Model file for the job. Use its own axes, mm. Face numbers are marked on the shaded views. A direction names the side the tool comes from. Coordinates: 2 decimals unless noted, no trailing zeros. Write each loop counter-clockwise with the first axis right and the second up, starting at its lowest first coordinate (ties: lowest second). Pieces come first, ordered by that corner, then holes.
Q1. Band-saw the part on D-D, the plane x = -7.55. Write the cut outline in (y, z) (3 decimals), plus the area to 3 significant figures.
Q2. Drill centre lines: probe 1 along Z at (x, y) = (-7.55, 17.25) (3 decimals); probe 2 along Z at (x, y) = (6.45, 26); probe 3 along X at (y, z) = (41.5, 45.6) (3 decimals). Where is each one in solid material? Low to high.
Q3. Which spindle directions (+Z, -Z, +X, -X, +Y, -Y) get a long thin tool onto all of the face, cutting with end or side? Do the marked faces 1, 2, 3 and 4. Say none if no direction does.
Q4. Pin check, flat tips, straight feed: P1, Ø16.5, axis at y = 27, z = 12, coming from the -X side; P2, Ø1.9, axis at y = 6, z = 31, coming from the -X side; P3, Ø4, axis at x = -7.55, z = 7, coming from the +Y side. Stop position of each tip, or through.
Q5. Band-saw the part on A-A, the plane x = 23. Write the cut outline in (y, z), plus the area to 3 significant figures.
Q6. Band-saw the part on B-B, the plane y = 26. Write the cut outline in (x, z) (3 decimals), plus the area to 3 significant figures.
Q7. Pull direction Z, two halves, no side cores. Call the marked faces 5, 6 and 7: released by +Z, released by -Z, zero draft, split by the parting line, or undercut.
from build123d import *

# Parameters (mm, degrees)
F0_W      = 10
F0_H      = 52
F1_DEPTH  = 44
F2_W      = 54
F2_H      = 52
F3_DEPTH  = 4
F5_DEPTH  = 4
F7_DEPTH  = 4
F8_R      = 15
F8_R_2    = 1.725
F9_DEPTH  = 4
F10_R     = 1.725
F11_DEPTH = 10
F10_R_2   = 3.5
F12_DEPTH = 6
F14_W     = 15.1
F14_H     = 4
F15_DEPTH = 48
F16_R     = 1.725
F17_DEPTH = 4
F18_R     = 1.725
F19_DEPTH = 4
F20_R     = 4
F21_R     = 1.99999


# Not quite as in the source:
# - a fillet or chamfer is up to 0.001 mm smaller than in the source, because OpenCascade refuses the exact size
# - a feature of the source that left no trace in its solid (it failed there, or was rolled back) is left out
# - a feature names something its author has since deleted; it is built from what else it names


with BuildPart() as f1:
    # F0 (on Top) → F1 (new body)
    with BuildSketch(Plane.XY):
        with Locations((5, 26)):
            Rectangle(F0_W, F0_H)
    extrude(amount=F1_DEPTH)

    # F2 (on face) → F3 (join)
    with BuildSketch(Plane.XY.offset(44)):
        with Locations((27, 26)):
            Rectangle(F2_W, F2_H)
    extrude(amount=F3_DEPTH)

    # F4 (on face) → F5 (join)
    with BuildSketch(Plane.XZ):
        Polygon((10, 0), (54, 44), (10, 44), align=None)
    extrude(amount=-F5_DEPTH)

    # F6 (on face) → F7 (join)
    with BuildSketch(Plane(origin=(0, 52, 0), x_dir=(-1, 0, 0), z_dir=(0, 1, 0))):
        Polygon((-10, 44), (-54, 44), (-10, 0), align=None)
    extrude(amount=-F7_DEPTH)

    # F8 (on face) → F9 (cut, through all)
    with BuildSketch(Plane(origin=(0, 0, 44), x_dir=(1, 0, 0), z_dir=(0, 0, -1))):
        with Locations((32, -26)):
            Circle(F8_R)
        with Locations((16.5, -10.5)):
            Circle(F8_R_2)
        with Locations((47.5, -10.5)):
            Circle(F8_R_2)
        with Locations((47.5, -41.5)):
            Circle(F8_R_2)
        with Locations((16.5, -41.5)):
            Circle(F8_R_2)
    extrude(amount=-F9_DEPTH, mode=Mode.SUBTRACT)

    # F10 (on face) → F11 (cut)
    with BuildSketch(Plane.YZ.offset(10)):
        with Locations((26, 37)):
            Circle(F10_R)
        with Locations((26, 7)):
            Circle(F10_R)
    extrude(amount=-F11_DEPTH, mode=Mode.SUBTRACT)

    # F10 (on face) → F12 (cut)
    with BuildSketch(Plane.YZ.offset(10)):
        with Locations((26, 37)):
            Circle(F10_R_2)
        with Locations((26, 37)):
            Circle(F10_R, mode=Mode.SUBTRACT)
        with Locations((26, 7)):
            Circle(F10_R_2)
        with Locations((26, 7)):
            Circle(F10_R, mode=Mode.SUBTRACT)
    extrude(amount=-F12_DEPTH, mode=Mode.SUBTRACT)

    # F14 (on face) → F15 (join)
    with BuildSketch(Plane.XY.offset(48)):
        with Locations((-7.55, 35.55)):
            Rectangle(F14_W, F14_H)
        with Locations((-7.55, 16.45)):
            Rectangle(F14_W, F14_H)
    extrude(amount=-F15_DEPTH)

    # F16 (on face) → F17 (cut, through all)
    with BuildSketch(Plane.XZ.offset(-14.45)):
        with Locations((-7.55, 37)):
            Circle(F16_R)
        with Locations((-7.55, 7)):
            Circle(F16_R)
    extrude(amount=-F17_DEPTH, mode=Mode.SUBTRACT)

    # F18 (on face) → F19 (cut, through all)
    with BuildSketch(Plane(origin=(0, 37.55, 0), x_dir=(-1, 0, 0), z_dir=(0, 1, 0))):
        with Locations((7.55, 37)):
            Circle(F18_R)
        with Locations((7.55, 7)):
            Circle(F18_R)
    extrude(amount=-F19_DEPTH, mode=Mode.SUBTRACT)

    # F20
    f20_edges = [f1.edges().sort_by_distance(p)[0] for p in [
        (0, 14.45, 24),
        (0, 37.55, 24),
        (0, 52, 24),
        (54, 52, 46),
        (54, 0, 46),
        (0, 0, 24),
    ]]
    fillet(f20_edges, radius=F20_R)

    # F21 (radius 2 in the source; OpenCascade refuses exactly that, so slightly less here)
    f21_edges = [f1.edges().sort_by_distance(p)[0] for p in [
        (-15.1, 37.55, 24),
        (-15.1, 33.55, 24),
        (-15.1, 18.45, 24),
        (-15.1, 14.45, 24),
    ]]
    fillet(f21_edges, radius=F21_R)


solid = f1.part
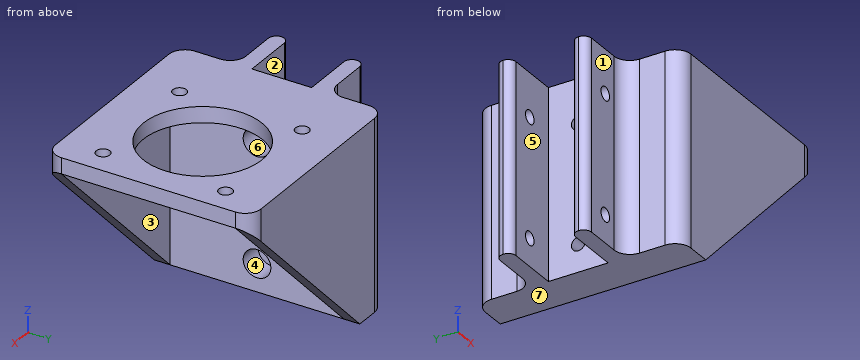
Answer sheet:
1. outline: (14.45, 0) - (18.45, 0) - (18.45, 5.275) - (14.45, 5.275) - close; (14.45, 8.725) - (18.45, 8.725) - (18.45, 35.275) - (14.45, 35.275) - close; (14.45, 38.725) - (18.45, 38.725) - (18.45, 48) - (14.45, 48) - close; (33.55, 0) - (37.55, 0) - (37.55, 5.275) - (33.55, 5.275) - close; (33.55, 8.725) - (37.55, 8.725) - (37.55, 35.275) - (33.55, 35.275) - close; (33.55, 38.725) - (37.55, 38.725) - (37.55, 48) - (33.55, 48) - close
1. area: 329 mm2
2. probe 1: z = 0 to 5.275, 8.725 to 35.275, 38.725 to 48
2. probe 2: z = 0 to 3.5, 10.5 to 33.5, 40.5 to 48
2. probe 3: x = 0 to 14.775, 18.225 to 45.775, 49.225 to 54
3. face 1: +Z, -Z, -X, -Y
3. face 2: +Z, -Z, -X
3. face 3: -Z, +X
3. face 4: +X
4. P1: stops at x = -15.08
4. P2: stops at x = 0
4. P3: stops at y = 37.55
5. outline: (0, 13) - (4, 13) - (4, 44) - (14, 44) - (14, 48) - (0, 48) - close; (38, 44) - (48, 44) - (48, 13) - (52, 13) - (52, 48) - (38, 48) - close
5. area: 360 mm2
6. outline: (0, 0) - (10, 0) - (10, 3.5) - (4, 3.5) - (4, 5.275) - (0, 5.275) - close; (0, 8.725) - (4, 8.725) - (4, 10.5) - (10, 10.5) - (10, 33.5) - (4, 33.5) - (4, 35.275) - (0, 35.275) - close; (0, 38.725) - (4, 38.725) - (4, 40.5) - (10, 40.5) - (10, 44) - (17, 44) - (17, 48) - (0, 48) - close; (47, 44) - (54, 44) - (54, 48) - (47, 48) - close
6. area: 424 mm2
7. face 5: zero draft
7. face 6: undercut
7. face 7: released by -Z
